Here's how the part is built. I have some questions about the finished solid (model axes, mm). A direction names the side the tool comes from. Round coordinates to 2 decimals unless told otherwise and drop trailing zeros. Write each loop counter-clockwise with the first axis right and the second up, starting at its lowest first coordinate (ties: lowest second). Pieces come first, ordered by that corner, then holes. Notation, with made-up numbers: (25.5, 6) -> (42.5, 6) arc R16 ccw to (42.5, 26) -> close; hole circle Ø1 at (46, 27). An arc over 180 degrees is marked (long way). Answer as CSV lines item,"result".
from build123d import *

# Parameters (mm, degrees)
BOSS_EXTRUDE1_DEPTH      = 12.7
SKETCH2_R                = 5
CUT_EXTRUDE1_DEPTH       = 33
SKETCH3_R                = 2.032
CUT_EXTRUDE2_DEPTH       = 7.62
CUT_EXTRUDE3_DEPTH       = 10.795
SKETCH5_R                = 1.5875
CUT_EXTRUDE4_DEPTH       = 10
SKETCH6_W                = 3.175
SKETCH6_H                = 11.169050429
CUT_EXTRUDE5_DEPTH       = 0.635
SKETCH7_R                = 6
CUT_EXTRUDE6_DEPTH       = 1.5494
SKETCH9_R                = 8.128
BOSS_EXTRUDE2_DEPTH      = 1.27
SKETCH10_R               = 6.35
CUT_EXTRUDE7_DEPTH       = 22.27
SKETCH11_R               = 1.143
CUT_EXTRUDE8_DEPTH       = 49.276
SKETCH12_R               = 1.143
CUT_EXTRUDE9_DEPTH       = 49.276
SKETCH13_R               = 1.143
CUT_EXTRUDE10_DEPTH      = 49.276
CUT_EXTRUDE11_DEPTH      = 50.8
CUT_EXTRUDE11_DEPTH_BACK = 50.8
SKETCH15_R               = 1.905


with BuildPart() as part:
    # Sketch1 → Boss-Extrude1 (new body)
    with BuildSketch(Plane.XY):
        with BuildLine():
            Line((-15.875, 246.311767937), (-15.875, 115.477708001))
            ThreePointArc((-15.875, 115.477708001), (-17.859739298, 101.416757728), (-23.658870968, 88.454520863))
            ThreePointArc((-23.658870968, 88.454520863), (-27.242596913, 67.388179182), (-14.890892485, 49.950597894))
            Line((-14.890892485, 49.950597894), (-4.737825133, 43.555823885))
            ThreePointArc((-4.737825133, 43.555823885), (0, 42.188131575), (4.737825135, 43.555823883))
            Line((4.737825135, 43.555823883), (14.890307558, 49.950229476))
            ThreePointArc((14.890307558, 49.950229476), (27.242520167, 67.387842169), (23.658870968, 88.454520863))
            ThreePointArc((23.658870968, 88.454520863), (17.859739298, 101.416757728), (15.875, 115.477708001))
            Line((15.875, 115.477708001), (15.875, 246.311767937))
            ThreePointArc((15.875, 246.311767937), (0, 262.186767937), (-15.875, 246.311767937))
        make_face()
    extrude(amount=BOSS_EXTRUDE1_DEPTH)

    # Sketch2 → Cut-Extrude1 (cut)
    with BuildSketch(Plane.XY.offset(12.7)):
        with Locations((0, 246.311767937)):
            Circle(SKETCH2_R)
    extrude(amount=-CUT_EXTRUDE1_DEPTH, mode=Mode.SUBTRACT)

    # Sketch3 → Cut-Extrude2 (cut)
    with BuildSketch(Plane.XY.offset(12.7)):
        with Locations((-8.89, 246.311767937)):
            Circle(SKETCH3_R)
        with Locations((-7.697390963, 250.754770656)):
            Circle(SKETCH3_R)
        with Locations((-4.443636151, 254.006796041)):
            Circle(SKETCH3_R)
        with Locations((0, 255.197042749)):
            Circle(SKETCH3_R)
        with Locations((4.443636151, 254.006796041)):
            Circle(SKETCH3_R)
        with Locations((7.697390963, 250.754770656)):
            Circle(SKETCH3_R)
        with Locations((8.89, 246.311767937)):
            Circle(SKETCH3_R)
    extrude(amount=-CUT_EXTRUDE2_DEPTH, mode=Mode.SUBTRACT)

    # Sketch4 → Cut-Extrude3 (cut)
    with BuildSketch(Plane.XY.offset(12.7)):
        with BuildLine():
            Line((-12.7, 238.691767937), (12.7, 238.691767937))
            ThreePointArc((12.7, 238.691767937), (13.598025612, 238.319793549), (13.97, 237.421767937))
            Line((13.97, 237.421767937), (13.97, 96.175375416))
            ThreePointArc((13.97, 96.175375416), (0, 47.036538193), (-13.97, 96.175375416))
            Line((-13.97, 96.175375416), (-13.97, 237.421767937))
            ThreePointArc((-13.97, 237.421767937), (-13.598025612, 238.319793549), (-12.7, 238.691767937))
        make_face()
    extrude(amount=-CUT_EXTRUDE3_DEPTH, mode=Mode.SUBTRACT)

    # Sketch5 → Cut-Extrude4 (cut)
    with BuildSketch(Plane.XY.offset(1.905)):
        with Locations((0, 235.311767937)):
            Circle(SKETCH5_R)
    extrude(amount=-CUT_EXTRUDE4_DEPTH, mode=Mode.SUBTRACT)

    # Sketch6 → Cut-Extrude5 (cut)
    with BuildSketch(Plane(origin=(0, 0, 0), x_dir=(-1, 0, 0), z_dir=(0, 0, -1))):
        with Locations((0, 240.896293152)):
            Rectangle(SKETCH6_W, SKETCH6_H)
    extrude(amount=-CUT_EXTRUDE5_DEPTH, mode=Mode.SUBTRACT)

    # Sketch7 → Cut-Extrude6 (cut)
    with BuildSketch(Plane(origin=(0, 0, 0), x_dir=(-1, 0, 0), z_dir=(0, 0, -1))):
        with Locations((0, 246.311767937)):
            Circle(SKETCH7_R)
    extrude(amount=-CUT_EXTRUDE6_DEPTH, mode=Mode.SUBTRACT)

    # Sketch9 → Boss-Extrude2 (add)
    with BuildSketch(Plane.XY.offset(1.905)):
        with Locations((0, 73.591767937)):
            Circle(SKETCH9_R)
    extrude(amount=BOSS_EXTRUDE2_DEPTH)

    # Sketch10 → Cut-Extrude7 (cut)
    with BuildSketch(Plane.XY.offset(3.175)):
        with Locations((0, 73.591767937)):
            Circle(SKETCH10_R)
    extrude(amount=-CUT_EXTRUDE7_DEPTH, mode=Mode.SUBTRACT)

    # Sketch11 → Cut-Extrude8 (cut)
    with BuildSketch(Plane.XY.offset(1.905)):
        with Locations((-10.4775, 101.709567937)):
            Circle(SKETCH11_R)
        with Locations((10.4775, 101.709567937)):
            Circle(SKETCH11_R)
    extrude(amount=-CUT_EXTRUDE8_DEPTH, mode=Mode.SUBTRACT)

    # Sketch12 → Cut-Extrude9 (cut)
    with BuildSketch(Plane.XY.offset(12.7)):
        with Locations((-16.764, 96.832767937)):
            Circle(SKETCH12_R)
        with Locations((16.764, 96.832767937)):
            Circle(SKETCH12_R)
        with Locations((0, 45.016767937)):
            Circle(SKETCH12_R)
    extrude(amount=-CUT_EXTRUDE9_DEPTH, mode=Mode.SUBTRACT)

    # Sketch13 → Cut-Extrude10 (cut)
    with BuildSketch(Plane.XY.offset(1.905)):
        with Locations((-6.35, 213.291767937)):
            Circle(SKETCH13_R)
        with Locations((6.35, 213.291767937)):
            Circle(SKETCH13_R)
        with Locations((-6.35, 137.091767937)):
            Circle(SKETCH13_R)
        with Locations((6.35, 137.091767937)):
            Circle(SKETCH13_R)
    extrude(amount=-CUT_EXTRUDE10_DEPTH, mode=Mode.SUBTRACT)

    # Sketch15 → Cut-Extrude11 (cut, two sides: drawn at the far end of the back side and taken through both)
    with BuildSketch(Plane.ZY.offset(-CUT_EXTRUDE11_DEPTH_BACK)):
        with Locations(Location((6.985, 73.591767937, 0), (0, 0, 90))):
            Circle(SKETCH15_R)
    extrude(amount=CUT_EXTRUDE11_DEPTH + CUT_EXTRUDE11_DEPTH_BACK, mode=Mode.SUBTRACT)


solid = part.part
Item 1: Suppose I cut it at A-A, the plane y = 182. List the corners of the cut face in (x, z) for me (3 decimals).
Results found:
outline,"(-15.875, 0) -> (15.875, 0) -> (15.875, 12.7) -> (13.97, 12.7) -> (13.97, 1.905) -> (-13.97, 1.905) -> (-13.97, 12.7) -> (-15.875, 12.7) -> close"
Item 2: If we mould it in two halves opening along X, with no side actions, what happens to faces 1 (the flat face through (14.4, 169, 12.7)), 2 (the flat face through (-9.89, 46.8, 6.26)), 3 (the flat face through (8, 251, 5.08))? For each: pulls with the +X half, pulls with the -X half, needs draft (parallel to the pull), parting line crosses it, or undercut.
Results found:
face 1,"needs draft"
face 2,"pulls with the -X half"
face 3,"undercut"
Item 3: Suppose I cut it at B-B, the plane x = 20.5. List the corners of the cut face in (y, z) for me (3 decimals), then the cut area to 3 significant figures.
Results found:
outline,"(54.608, 0) -> (94.3, 0) -> (94.3, 12.7) -> (90.472, 12.7) -> (90.472, 1.905) -> (56.712, 1.905) -> (56.712, 12.7) -> (54.608, 12.7) -> close"
area,"140 mm²"
Item 4: Will these pins go through, and if not, where does the flat tip stop? pin 1 (5 mm diameter, centred on x = 20, z = 7, fed in from -Y); pin 2 (11.5 mm diameter, centred on x = 0, y = 246.31, fed in from -Z); pin 3 (2 mm diameter, centred on x = 1.5, y = 112.5, fed in from +Z) (3 decimals).
Results found:
pin 1,"stops at y = 51.81"
pin 2,"stops at z = 1.55"
pin 3,"stops at z = 1.905"
Item 5: I need wall thicknesses on L1, parallel to X at y = 215.5, z = 2.75 (3 decimals); L2, parallel to Y at x = -9, z = 9; L3, parallel to Y at x = 7.5, z = 12.25. Which ranges of each line are inside material? Lowest first, please.
Results found:
L1,"x = -15.875 to -13.97, 13.97 to 15.875"
L2,"y = 46.24 to 48.61, 238.69 to 244.28, 248.34 to 249.2, 252.31 to 259.39"
L3,"y = 45.3 to 48.12, 238.69 to 244.83, 247.79 to 248.73, 252.78 to 260.3"
Item 6: For faces 4 (the flat face through (13.97, 168, 7)), 5 (the flat face through (4, 250, 1.549)), 6 (the cylindrical face through (-0.07, 42.19, 6.26)), which set-ups out of +Z, -Z, +X, -X, +Y, -Y let a thin tool reach every point of the face, with its end or its side?
Results found:
face 4,"+Z"
face 5,"-Z"
face 6,"+Z, -Z, -Y"
